Verification items for the finished model (mm, model axes). A direction names the side the tool comes from. Give positions to 0.01 mm unless a question says otherwise; leave off trailing zeros. Order: outer loops, then holes, each group sorted by start corner. A loop starts at its lowest first (then second) coordinate and runs counter-clockwise, first axis right, second up. Notation, with made-up numbers: (-15, 27.5) -> (28, 27.5) arc R14 ccw to (28, 48.5) -> close; hole circle Ø2 at (46, 34.5). An arc over 180 degrees is marked (long way). Write each question's results on one line, items separated by ' | '. Start each with the question number.
1. Cross-section at B-B, the plane y = 15.5. Enter the section's corners in (x, z) (3 decimals), then the cut area to 3 significant figures.
2. Cross-section at A-A, the plane y = 4.5. Enter the section's corners in (x, z) (3 decimals), then the cut area to 3 significant figures.
3. Mould release check, pull along Y, two halves, no side actions. Record for faces 1 (the face through (-15.497, 18.871, -3.441)), 2 (the face through (-13.22, 21.61, 1.74)), 3 (the face through (-0.05, 13.16, 8.53)): +Y half, -Y half, draft (parallel to the pull), parting line (faces both ways), or undercut.
4. Set-up check for faces 4 (the face through (0.7, 6.35, -1.4)), 5 (the face through (2.19, -6.44, -1.21)), 6 (the face through (-13, 20.32, 4)): record each of +Z, -Z, +X, -X, +Y, -Y from which the full face is reachable in a straight line by a thin tool's end or side.
5. Depth check by flat-ended pin: pin 1 Ø4 at (y, z) = (7, 5) entering from -X; pin 2 Ø3.5 at (y, z) = (7.5, 7) entering from -X; pin 3 Ø1.5 at (x, z) = (10.5, -6.5) entering from +Y. Enter the tip coordinate at first touch or a pass-through.
6. Material ranges on L1, parallel to Y at x = 8, z = -12; L2, parallel to Y at x = 11, z = -11; L3, parallel to Y at x = 6, z = 12, recorded low to high. Write a range as from..to.
7. Cross-section at D-D, the plane y = -7. Enter the section's corners in (x, z), then the cut area to 3 significant figures.
8. Cross-section at C-C, the plane y = 11.5. Enter the section's corners in (x, z) (3 decimals), then the cut area to 3 significant figures.
from build123d import *

# Parameters (mm, degrees)
SKETCH1_R           = 15.875
BOSS_EXTRUDE1_DEPTH = 25.4
SKETCH2_R           = 1.35
CUT_EXTRUDE2_DEPTH  = 25.4
CUT_EXTRUDE3_DEPTH  = 12.7
CUT_EXTRUDE5_DEPTH  = 39.885649667
SKETCH7_W           = 2.54
SKETCH7_H           = 2.54


with BuildPart() as part:
    # Sketch1 → Boss-Extrude1 (new body)
    with BuildSketch(Plane(origin=(0, 0, 0), x_dir=(1, 0, 0), z_dir=(0, 1, 0))):
        with Locations(Location((0, 0, 0), (0, 0, 270))):
            Circle(SKETCH1_R)
    extrude(amount=BOSS_EXTRUDE1_DEPTH)

    # Sketch2 → Cut-Extrude2 (cut)
    with BuildSketch(Plane(origin=(0, 25.4, 0), x_dir=(1, 0, 0), z_dir=(0, 1, 0))):
        with Locations(Location((0, 0, 0), (0, 0, 270))):
            Circle(SKETCH2_R)
    extrude(amount=-CUT_EXTRUDE2_DEPTH, mode=Mode.SUBTRACT)

    # Sketch3 → Revolve2 (revolve)
    with BuildSketch(Plane.XY):
        Polygon((0, 0), (0, -12.7), (-4.7625, -12.7), (-10.204772628, -3.2737073), (-15.875, 0), align=None)
    revolve(axis=Axis((0, 0, 0), (0, -1, 0)))

    # Sketch4 → Cut-Extrude3 (cut)
    with BuildSketch(Plane.XZ.offset(12.7)):
        with BuildLine():
            Line((1.412444273, -2.646696276), (2.987644573, 0.271992474))
            ThreePointArc((2.987644573, 0.271992474), (-2.640053308, 1.424822281), (1.412444273, -2.646696276))
        make_face()
    extrude(amount=-CUT_EXTRUDE3_DEPTH, mode=Mode.SUBTRACT)

    # Sketch5 → Cut-Revolve1 (revolve, cut)
    with BuildSketch(Plane.XY, mode=Mode.PRIVATE) as cut_revolve1_sk:
        Polygon((-12.065, 24.13), (-12.065, 19.05), (-6.35, 9.525), (-3.175, 9.525), (-3.175, 6.35), (0, 6.35), (0, 25.4), (-13.335, 25.4), align=None)
    revolve(cut_revolve1_sk.sketch.rotate(Axis((0, 6.35, 0), (0, 1, 0)), 270), axis=Axis((0, 6.35, 0), (0, 1, 0)), mode=Mode.SUBTRACT)

    # Sketch6 → Cut-Extrude5 (cut, through all)
    with BuildSketch(Plane(origin=(0, 19.05, 0), x_dir=(1, 0, 0), z_dir=(0, 1, 0))):
        with BuildLine():
            Line((-5.08, 0), (-11.484424543, 3.697596234))
            ThreePointArc((-11.484424543, 3.697596234), (-12.065, 0), (-11.484424543, -3.697596234))
            Line((-11.484424543, -3.697596234), (-5.08, 0))
        make_face()
        with BuildLine():
            Line((-2.54, 4.399409051), (-2.54, 11.794601519))
            ThreePointArc((-2.54, 11.794601519), (-6.0325, 10.448596497), (-8.944424543, 8.097005285))
            Line((-8.944424543, 8.097005285), (-2.54, 4.399409051))
        make_face()
        with BuildLine():
            Line((2.54, 4.399409051), (8.944424543, 8.097005285))
            ThreePointArc((8.944424543, 8.097005285), (6.0325, 10.448596497), (2.54, 11.794601519))
            Line((2.54, 11.794601519), (2.54, 4.399409051))
        make_face()
        with BuildLine():
            Line((5.08, 0), (11.484424543, -3.697596234))
            ThreePointArc((11.484424543, -3.697596234), (12.065, 0), (11.484424543, 3.697596234))
            Line((11.484424543, 3.697596234), (5.08, 0))
        make_face()
        with BuildLine():
            Line((2.54, -4.399409051), (2.54, -11.794601519))
            ThreePointArc((2.54, -11.794601519), (6.0325, -10.448596497), (8.944424543, -8.097005285))
            Line((8.944424543, -8.097005285), (2.54, -4.399409051))
        make_face()
        with BuildLine():
            Line((-8.944424543, -8.097005285), (-2.54, -4.399409051))
            Line((-2.54, -4.399409051), (-2.54, -11.794601519))
            ThreePointArc((-2.54, -11.794601519), (-6.0325, -10.448596497), (-8.944424543, -8.097005285))
        make_face()
    extrude(amount=-CUT_EXTRUDE5_DEPTH, mode=Mode.SUBTRACT)

    # Sketch7 → Cut-Revolve2 (revolve, cut)
    with BuildSketch(Plane.XY, mode=Mode.PRIVATE) as cut_revolve2_sk:
        with Locations((-14.605, 21.59)):
            Rectangle(SKETCH7_W, SKETCH7_H)
        with Locations((-14.605, 3.81)):
            Rectangle(SKETCH7_W, SKETCH7_H)
        Polygon((-15.875, 17.4625), (-15.875, 7.9375), (-14.605, 9.2075), (-14.605, 16.1925), align=None)
    revolve(cut_revolve2_sk.sketch.rotate(Axis((0, 0, 0), (0, 1, 0)), 270), axis=Axis((0, 0, 0), (0, 1, 0)), mode=Mode.SUBTRACT)


solid = part.part
Results below:
1) outline: circle Ø29.21 at (0, 0); hole (-11.484, -3.698) -> (-9.588, -2.603) arc R9.935 ccw to (-7.048, -7.002) -> (-8.944, -8.097) arc R12.065 ccw to (-2.54, -11.795) -> (-2.54, -9.605) arc R9.935 ccw to (2.54, -9.605) -> (2.54, -11.795) arc R12.065 ccw to (8.944, -8.097) -> (7.048, -7.002) arc R9.935 ccw to (9.588, -2.603) -> (11.484, -3.698) arc R12.065 ccw to (11.484, 3.698) -> (9.588, 2.603) arc R9.935 ccw to (7.048, 7.002) -> (8.944, 8.097) arc R12.065 ccw to (2.54, 11.795) -> (2.54, 9.605) arc R9.935 ccw to (-2.54, 9.605) -> (-2.54, 11.795) arc R12.065 ccw to (-8.944, 8.097) -> (-7.048, 7.002) arc R9.935 ccw to (-9.588, 2.603) -> (-11.484, 3.698) arc R12.065 ccw to start | area: 278 mm²
2) outline: circle Ø26.67 at (0, 0); hole (-11.484, -3.698) -> (-5.08, 0) -> (-11.484, 3.698) arc R12.065 ccw to start; hole (-8.944, -8.097) arc R12.065 ccw to (-2.54, -11.795) -> (-2.54, -4.399) -> close; hole (-8.944, 8.097) -> (-2.54, 4.399) -> (-2.54, 11.795) arc R12.065 ccw to start; hole circle Ø2.7 at (0, 0); hole (2.54, -11.795) arc R12.065 ccw to (8.944, -8.097) -> (2.54, -4.399) -> close; hole (2.54, 4.399) -> (8.944, 8.097) arc R12.065 ccw to (2.54, 11.795) -> close; hole (5.08, 0) -> (11.484, -3.698) arc R12.065 ccw to (11.484, 3.698) -> close | area: 394 mm²
3) face 1: draft | face 2: undercut | face 3: +Y half
4) face 4: +Y | face 5: -Y | face 6: none
5) pin 1: stops at x = -15.59 | pin 2: stops at x = -14.98 | pin 3: stops at y = 25.16
6) L1: y = -0.84..2.54, 5.08..20.32, 22.86..25.4 | L2: y = -0.18..2.54, 5.08..8.26, 17.14..20.32, 22.86..25.4 | L3: y = -1.42..2.54, 5.08..20.32, 22.86..25.4
7) outline: (-7.89, -1.62) arc R8.05 ccw to (-5.35, -6.02) -> (-2.54, -4.4) -> (-2.54, -7.64) arc R8.05 ccw to (2.54, -7.64) -> (2.54, -4.4) -> (5.35, -6.02) arc R8.05 ccw to (7.89, -1.62) -> (5.08, 0) -> (7.89, 1.62) arc R8.05 ccw to (5.35, 6.02) -> (2.54, 4.4) -> (2.54, 7.64) arc R8.05 ccw to (-2.54, 7.64) -> (-2.54, 4.4) -> (-5.35, 6.02) arc R8.05 ccw to (-7.89, 1.62) -> (-5.08, 0) -> close; hole (1.41, -2.65) -> (2.99, 0.27) arc R3 ccw (long way) to start | area: 147 mm²
8) outline: circle Ø29.21 at (0, 0); hole (-11.484, -3.698) -> (-7.414, -1.347) arc R7.535 ccw to (-4.874, -5.747) -> (-8.944, -8.097) arc R12.065 ccw to (-2.54, -11.795) -> (-2.54, -7.094) arc R7.535 ccw to (2.54, -7.094) -> (2.54, -11.795) arc R12.065 ccw to (8.944, -8.097) -> (4.874, -5.747) arc R7.535 ccw to (7.414, -1.347) -> (11.484, -3.698) arc R12.065 ccw to (11.484, 3.698) -> (7.414, 1.347) arc R7.535 ccw to (4.874, 5.747) -> (8.944, 8.097) arc R12.065 ccw to (2.54, 11.795) -> (2.54, 7.094) arc R7.535 ccw to (-2.54, 7.094) -> (-2.54, 11.795) arc R12.065 ccw to (-8.944, 8.097) -> (-4.874, 5.747) arc R7.535 ccw to (-7.414, 1.347) -> (-11.484, 3.698) arc R12.065 ccw to start | area: 353 mm²
